For this review, take the finished solid that the model builds, in its own axes (mm). A direction names the side the tool comes from. Round coordinates to 2 decimals unless told otherwise and drop trailing zeros. Order: outer loops, then holes, each group sorted by start corner. A loop starts at its lowest first (then second) coordinate and runs counter-clockwise, first axis right, second up. Notation, with made-up numbers: M 35.25,80.5 L 48.25,80.5 A23 cw 48.25,105.5 Z; hole C 39.25,61.25 d10. An arc over 180 degrees is marked long. Answer in a Markdown table with one row per item. Add a question column.
```python
from build123d import *

# Parameters (mm, degrees)
SKETCH1_R           = 5
BOSS_EXTRUDE1_DEPTH = 8
SKETCH2_W           = 12
SKETCH2_H           = 11
BOSS_EXTRUDE2_DEPTH = 10


with BuildPart() as part:
    # Sketch1 → Boss-Extrude1 (new body)
    with BuildSketch(Plane.XY):
        Circle(SKETCH1_R)
    extrude(amount=BOSS_EXTRUDE1_DEPTH)

    # Sketch2 → Boss-Extrude2 (add)
    with BuildSketch(Plane.XY.offset(8)):
        Rectangle(SKETCH2_W, SKETCH2_H)
    extrude(amount=BOSS_EXTRUDE2_DEPTH)

    # Sketch3 → Loft1 section 0
    with BuildSketch(Plane(origin=(0, 0, 8), x_dir=(-1, 0, 0), z_dir=(0, 0, -1))):
        with BuildLine():
            Line((6, -5.5), (6, 5.5))
            Line((6, 5.5), (-6, 5.5))
            Line((-6, 5.5), (-6, -5.5))
            Line((-6, -5.5), (6, -5.5))
        make_face()
    # Sketch4 → Loft1 section 1
    with BuildSketch(Plane.XY.offset(18)):
        with BuildLine():
            Line((7.25, -5.75), (-7.25, -5.75))
            Line((-7.25, -5.75), (-7.25, 5.75))
            Line((-7.25, 5.75), (7.25, 5.75))
            Line((7.25, 5.75), (7.25, -5.75))
        make_face()
    loft()


solid = part.part
```
1. Clearance check with flat-ended pins moving along their axes: pin 1 Ø6 at (y, z) = (4.5, 2.5) entering from +X; pin 2 Ø1 at (y, z) = (0.5, 4) entering from +X; pin 3 Ø8 at (x, z) = (-4, 2) entering from -Y. State where each tip first meets the part, or that it passes through.
2. For faces 1 (the cylindrical face through (-1.08, -4.88, 3.94)), 2 (the flat face through (0, 0, 18)), list the 3-axis set-ups (+Z, -Z, +X, -X, +Y, -Y) from which the entire face can be reached by the end or side of a thin tool; tool diameter is ignored.
3. Consider section A-A on z = 5. Write out the cut boundary in (x, y).
4. To check wall thickness, follow probe 1 along Z at (x, y) = (2.25, -4.75); probe 2 along X at (y, z) = (4, 10.25); probe 3 along X at (y, z) = (0, 9.5). State the ranges of each line that lie inside material, in increasing order. Write a range as [from, to].
Solved:
| question | item | result |
|---|---|---|
| 1 | pin 1 | stops at x = 4.77 |
| 1 | pin 2 | stops at x = 5 |
| 1 | pin 3 | stops at y = -5 |
| 2 | face 1 | -Z |
| 2 | face 2 | +Z, +X, -X, +Y, -Y |
| 3 | outline | C 0,0 d10 |
| 4 | probe 1 | z = [8, 18] |
| 4 | probe 2 | x = [-6.28, 6.28] |
| 4 | probe 3 | x = [-6.19, 6.19] |
